```python
from build123d import *

# Parameters (mm, degrees)
SKETCH1_W           = 9.8
SKETCH1_H           = 6.8
BOSS_EXTRUDE1_DEPTH = 4.7
SKETCH2_W           = 11
SKETCH2_H           = 8
BOSS_EXTRUDE2_DEPTH = 0.5
SKETCH3_W           = 8
SKETCH3_H           = 5
CUT_EXTRUDE1_DEPTH  = 3.7
FILLET1_R           = 0.5


with BuildPart() as part:
    # Sketch1 → Boss-Extrude1 (new body)
    with BuildSketch(Plane(origin=(0, 0, 0), x_dir=(1, 0, 0), z_dir=(0, 1, 0))):
        with Locations((4.9, 3.4)):
            Rectangle(SKETCH1_W, SKETCH1_H)
    extrude(amount=BOSS_EXTRUDE1_DEPTH)

    # Sketch2 → Boss-Extrude2 (add)
    with BuildSketch(Plane.XZ):
        with Locations((4.9, -3.4)):
            Rectangle(SKETCH2_W, SKETCH2_H)
    extrude(amount=BOSS_EXTRUDE2_DEPTH)

    # Sketch3 → Cut-Extrude1 (cut)
    with BuildSketch(Plane.XZ.offset(0.5)):
        with Locations((4.9, -3.4)):
            Rectangle(SKETCH3_W, SKETCH3_H)
    extrude(amount=-CUT_EXTRUDE1_DEPTH, mode=Mode.SUBTRACT)

    # Fillet1
    fillet1_edges = [part.edges().sort_by_distance(p)[0] for p in [
        (0, 2.35, -6.8),
        (9.8, 2.35, -6.8),
        (9.8, 2.35, 0),
        (0, 2.35, 0),
    ]]
    fillet(fillet1_edges, radius=FILLET1_R)


solid = part.part
```
Work out the finished part from the listing and answer in its coordinate system (mm). A direction names the side the tool comes from. Coordinates: 2 decimals unless noted, no trailing zeros. Write each loop counter-clockwise with the first axis right and the second up, starting at its lowest first coordinate (ties: lowest second). Pieces come first, ordered by that corner, then holes. Notation, with made-up numbers: (-19.75, 43) - (-14.75, 43) arc R21 cw to (-14.75, 80) - close; hole circle Ø1 at (70, -10.75). An arc over 180 degrees is marked (long way). Answer as a JSON object with one key per item and string values.
Q1. Find section B-B (x = 8.5). Write down the section's boundary in (y, z), plus the area to 3 significant figures.
Results list:
{"outline": "(-0.5, -7.4) - (0, -7.4) - (0, -6.8) - (4.7, -6.8) - (4.7, 0) - (0, 0) - (0, 0.6) - (-0.5, 0.6) - (-0.5, -0.9) - (3.2, -0.9) - (3.2, -5.9) - (-0.5, -5.9) - close", "area": "17.5 mm^2"}
Q2. Given pin 1 Ø2 at (y, z) = (2, -5) entering from +X; pin 2 Ø1 at (x, y) = (1.5, 1) entering from +Z; pin 3 Ø2.5 at (x, z) = (6, -3.5) entering from -Y, each flat-ended and moving along its own axis, determine where each tip first touches the part or whether it passes through.
Results list:
{"pin 1": "stops at x = 9.8", "pin 2": "stops at z = 0", "pin 3": "stops at y = 3.2"}
Q3. For a pull along Z with two mould halves and no side action, classify faces 1 (the flat face through (5, 2, 0)), 2 (the flat face through (5, 3.2, -3)), 3 (the flat face through (5, 1, -5.9)), 4 (the flat face through (5, 2, -6.8)) as pulls with the +Z half, pulls with the -Z half, needs draft (parallel to the pull), parting line crosses it, or undercut.
Results list:
{"face 1": "pulls with the +Z half", "face 2": "undercut", "face 3": "undercut", "face 4": "pulls with the -Z half"}
Q4. Find section A-A (y = 2.4). Write down the section's boundary in (x, z).
Results list:
{"outline": "(0, -6.3) arc R0.5 ccw to (0.5, -6.8) - (9.3, -6.8) arc R0.5 ccw to (9.8, -6.3) - (9.8, -0.5) arc R0.5 ccw to (9.3, 0) - (0.5, 0) arc R0.5 ccw to (0, -0.5) - close; hole (0.9, -5.9) - (8.9, -5.9) - (8.9, -0.9) - (0.9, -0.9) - close"}
Q5. Find section C-C (z = -5.75). Write down the section's boundary in (x, y).
Results list:
{"outline": "(-0.6, -0.5) - (0.9, -0.5) - (0.9, 3.2) - (8.9, 3.2) - (8.9, -0.5) - (10.4, -0.5) - (10.4, 0) - (9.8, 0) - (9.8, 4.7) - (0, 4.7) - (0, 0) - (-0.6, 0) - close"}
Q6. Which of the six approach directions +Z, -Z, +X, -X, +Y, -Y give full straight-line access (tool end or side, diameter ignored) to faces 5 (the flat face through (8.9, 1, -3)), 6 (the flat face through (0, 2, -3)), 7 (the flat face through (9.8, 2, -3))?
Results list:
{"face 5": "-Y", "face 6": "+Z, -Z, -X, +Y", "face 7": "+Z, -Z, +X, +Y"}
Q7. Find section D-D (y = 3.9). Write down the section's boundary in (x, z).
Results list:
{"outline": "(0, -6.3) arc R0.5 ccw to (0.5, -6.8) - (9.3, -6.8) arc R0.5 ccw to (9.8, -6.3) - (9.8, -0.5) arc R0.5 ccw to (9.3, 0) - (0.5, 0) arc R0.5 ccw to (0, -0.5) - close"}
Q8. Consider L1, parallel to X at y = 1, z = -2; L2, parallel to Z at x = 5, y = 0.75; L3, parallel to Z at x = 0.5, y = 0.25. Determine where each line is inside the solid, lowest interval first. Write a range as from..to.
Results list:
{"L1": "x = 0..0.9, 8.9..9.8", "L2": "z = -6.8..-5.9, -0.9..0", "L3": "z = -6.8..0"}
